from build123d import *

# Parameters (mm, degrees)
BOSS_EXTRUDE1_DEPTH = 21
CIRPATTERN1_COUNT   = 4
CUT_EXTRUDE2_DEPTH  = 46
SKETCH12_W          = 3.4
SKETCH12_H          = 35
CIRPATTERN2_COUNT   = 2
CIRPATTERN2_ANGLE   = 90


with BuildPart() as part:
    # Sketch3 → Revolve2 (revolve)
    with BuildSketch(Plane(origin=(0, 0, 0), x_dir=(0, 0, -1), z_dir=(1, 0, 0))):
        Polygon((22.5, 0), (22.5, 34.5), (22, 35), (-0.5, 35), (-0.5, 39.5), (-1, 40), (-22.5, 40), (-22.5, 0), align=None)
    revolve(axis=Axis((0, 0, 22.5), (0, 0, -1)))

    # Sketch5 → Boss-Extrude1 (add)
    with BuildSketch(Plane.XY.offset(22.5)):
        with BuildLine():
            Line((-4.365, 23.59972), (-10.56935, 38.578347))
            ThreePointArc((-10.56935, 38.578347), (0, 40), (10.56935, 38.578347))
            Line((10.56935, 38.578347), (4.365, 23.59972))
            ThreePointArc((4.365, 23.59972), (0, 24), (-4.365, 23.59972))
        make_face()
    boss_extrude1 = extrude(amount=BOSS_EXTRUDE1_DEPTH)

    # CirPattern1: Boss-Extrude1 ×4 about axis
    cirpattern1_axis = Axis((0, 0, 0), (0, 0, 1))
    for i in range(1, CIRPATTERN1_COUNT):
        add(boss_extrude1.rotate(cirpattern1_axis, i * 360 / CIRPATTERN1_COUNT))

    # Sketch6 → Cut-Extrude2 (cut, through all)
    with BuildSketch(Plane.XY.offset(22.5)):
        with BuildLine():
            ThreePointArc((12, 0), (2.029224, 11.827183), (-11.313708, 4))
            Line((-11.313708, 4), (-8.7, 4))
            Line((-8.7, 4), (-8.7, -4))
            Line((-8.7, -4), (-11.313708, -4))
            ThreePointArc((-11.313708, -4), (2.029224, -11.827183), (12, 0))
        make_face()
        with BuildLine():
            Line((-8.7, 4), (-11.313708, 4))
            ThreePointArc((-11.313708, 4), (-12, 0), (-11.313708, -4))
            Line((-11.313708, -4), (-8.7, -4))
            Line((-8.7, -4), (-8.7, 4))
        make_face()
        with BuildLine():
            Line((-11.313708, 4), (-15.3, 4))
            Line((-15.3, 4), (-15.3, -4))
            Line((-15.3, -4), (-11.313708, -4))
            ThreePointArc((-11.313708, -4), (-12, 0), (-11.313708, 4))
        make_face()
    extrude(amount=-CUT_EXTRUDE2_DEPTH, mode=Mode.SUBTRACT)

    # Sketch12 → Tap Drill for M8x1.25 Tap2 (revolve, cut)
    with BuildSketch(Plane(origin=(0, 0, -12.5), x_dir=(0, 0, 1), z_dir=(0, 1, 0))):
        with Locations((1.7, 17.5)):
            Rectangle(SKETCH12_W, SKETCH12_H)
    tap_drill_for_m8x1_25_tap2 = revolve(axis=Axis((-6.35, 0, -12.5), (1, 0, 0)), mode=Mode.SUBTRACT)

    # CirPattern2: Tap Drill for M8x1.25 Tap2 ×2 about axis
    cirpattern2_axis = Axis((0, 0, 22.5), (0, 0, 1))
    for i in range(1, CIRPATTERN2_COUNT):
        add(tap_drill_for_m8x1_25_tap2.rotate(cirpattern2_axis, i * CIRPATTERN2_ANGLE / (CIRPATTERN2_COUNT - 1)), mode=Mode.SUBTRACT)


solid = part.part
Can you work these out from the model? Positions are in its coordinate system, mm. A direction names the side the tool comes from. Round coordinates to 2 decimals unless told otherwise and drop trailing zeros. Loops run counter-clockwise (first coordinate to the right, second up) from the corner with the lowest first, then second, coordinate; pieces in that order, holes last. Notation, with made-up numbers: (31.25, -20) - (61.25, -20) arc R10 ccw to (61.25, -9) - close; hole circle Ø11 at (86, 23.25). An arc over 180 degrees is marked (long way). Use CSV: the item, a comma, the result in double quotes. Start each with the question number.
1) For pin 1 Ø2 at (x, z) = (-9, 14.5) entering from +Y; pin 2 Ø4 at (x, z) = (24, -15.5) entering from -Y; pin 3 Ø2 at (x, z) = (-10.5, 34) entering from +Y, each with a flat end and sliding along its axis, tell me the tip position at first contact or that it passes through.
2) For faces 1 (the cylindrical face through (-21, -28, -11)), 2 (the flat face through (-13, -4, 0)), 3 (the cylindrical face through (0, -24, 33)), 4 (the flat face through (-7.51, -31.19, 32.85)), which set-ups out of +Z, -Z, +X, -X, +Y, -Y let a thin tool reach every point of the face, with its end or its side?
3) Please list where these lines run through material, in increasing order: probe 1 along X at (y, z) = (-0.5, -20); probe 2 along Z at (x, y) = (29, 0); probe 3 along Z at (x, y) = (16.75, 0). Write a range as [from, to].
4) If we section it at B-B on z = 33.5: Write out the boundary of the cut face in (x, y) (3 decimals), plus the area to 3 significant figures.
5) We'd pull the mould along Y, two halves only. Please class faces 5 (the flat face through (-26, 24, 0.5)), 6 (the flat face through (31.19, -7.51, 32.85)), 7 (the cylindrical face through (23.419, 2.069, -15.198)), 8 (the flat face through (7.42, -30.98, 32.85)): released by +Y, released by -Y, zero draft, split by the parting line, or undercut.
6) If we section it at C-C on z = -17.5: Write out the boundary of the cut face in (x, y).
7) If we section it at A-A on x = 0: Write out the boundary of the cut face in (y, z), plus the area to 3 significant figures.
Geometry results:
1,pin 1,"stops at y = 39.19"
1,pin 2,"stops at y = -27.22"
1,pin 3,"stops at y = 38.86"
2,face 1,"-Z"
2,face 2,"+Z, -Z"
2,face 3,"+Z"
2,face 4,"+Z, -X"
3,probe 1,"x = [-35, -15.3], [11.99, 35]"
3,probe 2,"z = [-22.5, -15.9], [-9.1, 43.5]"
3,probe 3,"z = [-22.5, -15.9], [-9.1, 22.5]"
4,outline,"(-38.578, -10.569) - (-23.6, -4.365) arc R24 cw to (-23.6, 4.365) - (-38.578, 10.569) arc R40 ccw to start; (-10.569, -38.578) arc R40 ccw to (10.569, -38.578) - (4.365, -23.6) arc R24 cw to (-4.365, -23.6) - close; (-10.569, 38.578) - (-4.365, 23.6) arc R24 cw to (4.365, 23.6) - (10.569, 38.578) arc R40 ccw to start; (23.6, -4.365) - (38.578, -10.569) arc R40 ccw to (38.578, 10.569) - (23.6, 4.365) arc R24 cw to start"
4,area,"966 mm2"
5,face 5,"zero draft"
5,face 6,"released by -Y"
5,face 7,"undercut"
5,face 8,"undercut"
6,outline,"circle Ø70 at (0, 0); hole (-15.3, -4) - (-11.31, -4) arc R12 ccw to (12, 0) arc R12 ccw to (-11.31, 4) - (-15.3, 4) - close"
7,outline,"(-40, 1) - (-39.5, 0.5) - (-35, 0.5) - (-35, -22) - (-34.5, -22.5) - (-12, -22.5) - (-12, 22.5) - (-24, 22.5) - (-24, 43.5) - (-40, 43.5) - close; (12, -22.5) - (34.5, -22.5) - (35, -22) - (35, -15.9) - (12, -15.9) - close; (12, -9.1) - (35, -9.1) - (35, 0.5) - (39.5, 0.5) - (40, 1) - (40, 43.5) - (24, 43.5) - (24, 22.5) - (12, 22.5) - close"
7,area,"2,810 mm2"
